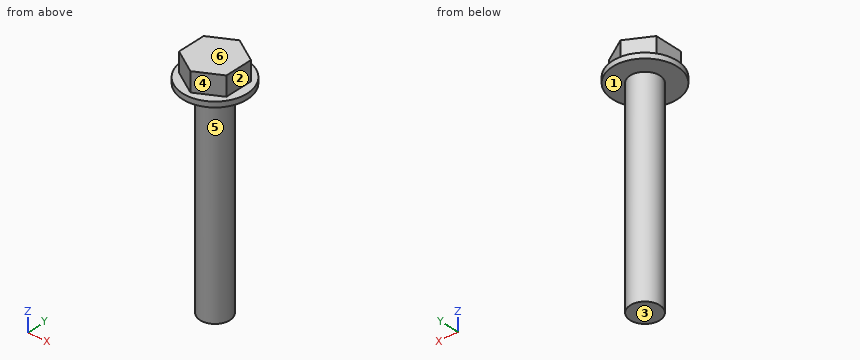
from build123d import *

# Parameters (mm, degrees)
EXTRUDE_SKETCH_1_R = 10.92
EXTRUDE_1_DEPTH    = 1.8
EXTRUDE_START      = 1.8
EXTRUDE_2_DEPTH    = 6.5
EXTRUDE_START_2    = -70
EXTRUDE_SKETCH_3_R = 5
EXTRUDE_3_DEPTH    = 70.01


with BuildPart() as part:
    # Extrude sketch 1 → Extrude 1 (new body)
    with BuildSketch(Plane.XY):
        Circle(EXTRUDE_SKETCH_1_R)
    extrude(amount=EXTRUDE_1_DEPTH)


with BuildPart() as body_2:
    # Extrude sketch 2 → Extrude 2 (new body)
    with BuildSketch(Plane.XY.offset(EXTRUDE_START)):
        Polygon((8, 4.618802154), (0, 9.237604307), (-8, 4.618802154), (-8, -4.618802154), (0, -9.237604307), (8, -4.618802154), align=None)
    extrude(amount=EXTRUDE_2_DEPTH)


with BuildPart() as body_3:
    # Extrude sketch 3 → Extrude 3 (new body)
    with BuildSketch(Plane.XY.offset(EXTRUDE_START_2)):
        Circle(EXTRUDE_SKETCH_3_R)
    extrude(amount=EXTRUDE_3_DEPTH)


with BuildPart() as part_1:
    add(part.part)

    # Combine (weld / assembly of features): union body 3, body 2
    add(body_3.part)
    add(body_2.part)


solid = part_1.part
Source: CAD feature listing. Evaluate the final solid. Frame: model axes, mm. Face numbers are marked on the shaded views. A direction names the side the tool comes from. Give positions to 0.01 mm unless a question says otherwise; leave off trailing zeros. Write each loop counter-clockwise with the first axis right and the second up, starting at its lowest first coordinate (ties: lowest second). Pieces come first, ordered by that corner, then holes. Notation, with made-up numbers: M -33.5,28 L -7.5,28 A14 ccw -7.5,42 Z; hole C 64.5,9.5 d1. An arc over 180 degrees is marked long. Return JSON: item names as keys, results as strings. Group by question number.
1) Cut plane B-B, the plane x = -3. Output: boundary loops of the cut face in (y, z), plus the area to 3 significant figures.
2) Cut plane C-C, the plane z = -51. Output: boundary loops of the cut face in (x, y).
3) Pull-direction query (X, two-part tool) for the marked faces 4, 5 and 6; classes: pulls with the +X half, pulls with the -X half, needs draft (parallel to the pull), parting line crosses it, or undercut.
4) Pin query (flat end, axial travel): P1, Ø3, axis at y = 2.5, z = -32, coming from the +X side; P2, Ø7, axis at y = -2, z = 6.5, coming from the -X side; P3, Ø1, axis at y = -2.5, z = -47, coming from the +X side. Return the tip coordinate at first contact, or that it passes through.
5) Material intervals for line 1 along Y through (x, z) = (0.25, -36); line 2 along Z through (x, y) = (-5.75, 0.75); line 3 along Z through (x, y) = (8.5, 3), sorted ascending. Write a range as [from, to].
6) Cut plane A-A, the plane y = 0. Output: boundary loops of the cut face in (x, z).
7) Cut plane D-D, the plane x = 6.5. Output: boundary loops of the cut face in (y, z).
8) Set-up query: the marked faces 1, 2 and 3. Return all of +Z, -Z, +X, -X, +Y, -Y with unobstructed straight access to the full face (end or side cutting, diameter ignored); none if empty.
Recorded:
{
 "1": {"outline": "M -10.5,0 L -4,0 L -4,-70 L 4,-70 L 4,0 L 10.5,0 L 10.5,1.8 L 7.51,1.8 L 7.51,8.3 L -7.51,8.3 L -7.51,1.8 L -10.5,1.8 Z", "area": "695 mm²"},
 "2": {"outline": "C 0,0 d10"},
 "3": {"face 4": "pulls with the +X half", "face 5": "parting line crosses it", "face 6": "needs draft"},
 "4": {"P1": "stops at x = 4.9", "P2": "stops at x = -8", "P3": "stops at x = 4.58"},
 "5": {"line 1": "y = [-4.99, 4.99]", "line 2": "z = [0, 8.3]", "line 3": "z = [0, 1.8]"},
 "6": {"outline": "M -10.92,0 L -5,0 L -5,-70 L 5,-70 L 5,0 L 10.92,0 L 10.92,1.8 L 8,1.8 L 8,8.3 L -8,8.3 L -8,1.8 L -10.92,1.8 Z"},
 "7": {"outline": "M -8.77,0 L 8.77,0 L 8.77,1.8 L 5.48,1.8 L 5.48,8.3 L -5.48,8.3 L -5.48,1.8 L -8.77,1.8 Z"},
 "8": {"face 1": "-Z", "face 2": "+Z, +X, +Y, -Y", "face 3": "-Z, +X, -X, +Y, -Y"}
}
